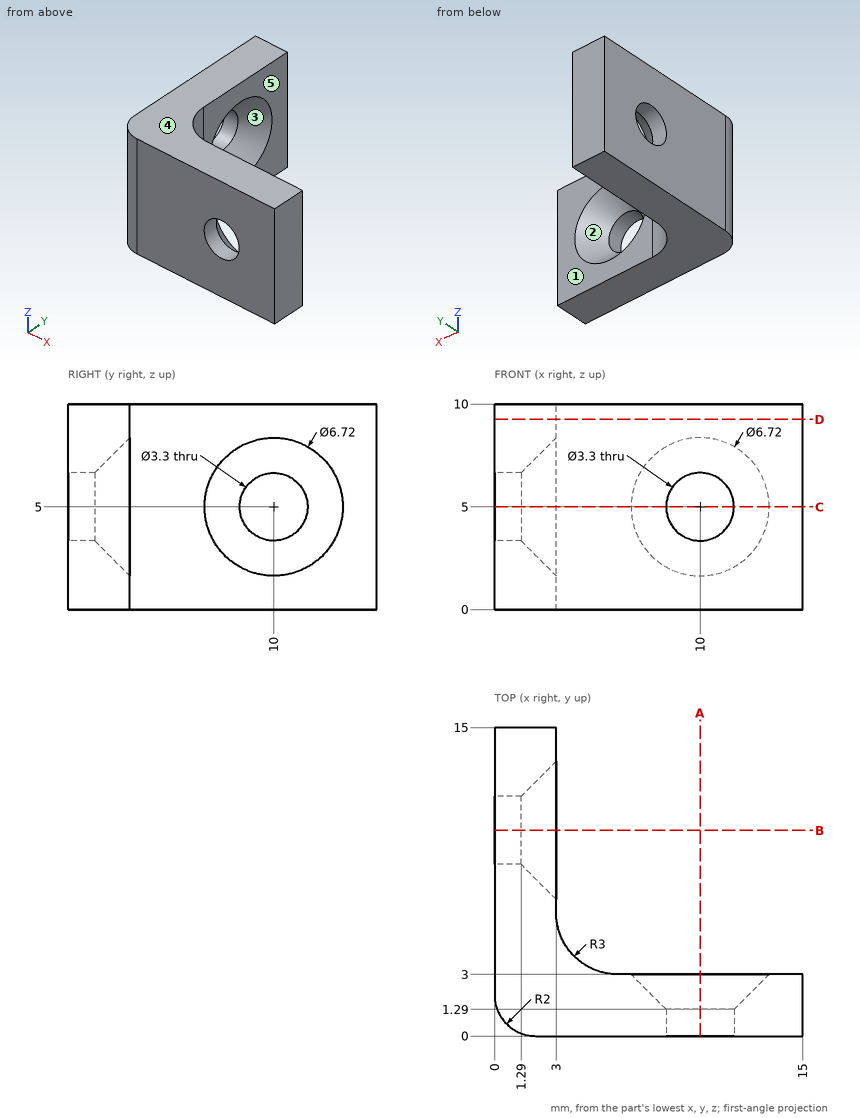
Job drawing, mm, ordinate dimensions from the low corner. One solid piece. A direction names the side the tool comes from. Coordinates: 2 decimals unless noted, no trailing zeros. Loops run counter-clockwise (first coordinate to the right, second up) from the corner with the lowest first, then second, coordinate; pieces in that order, holes last. Notation, with made-up numbers: (53.5, 47) - (100.5, 47) arc R15 ccw to (100.5, 52) - close; hole circle Ø3 at (46.25, 10). An arc over 180 degrees is marked (long way). Answer as a JSON object with one key per item and string values. Group by question number.
(1) Cut at A-A (x = 10). Give the cut face in (y, z), then the cut area to 3 significant figures.
(2) Cut at C-C (z = 5). Give the cut face in (x, y), then the cut area to 3 significant figures.
(3) Tool access for the marked faces 1 and 2: list every direction of +Z, -Z, +X, -X, +Y, -Y with a clear straight run to the whole face (end or side of a thin tool).
(4) Probe line 1 along Z through (x, y) = (10, 0.6); line 2 along X through (y, z) = (8.75, 7); line 3 along Y through (x, z) = (0.3, 5). List the from-to ranges inside material, lowest first.
(5) Cut at D-D (z = 9.25). Give the cut face in (x, y).
(6) Two-plate mould, pull along Z, no slides. Class the marked faces 3, 4 and 5: released by +Z, released by -Z, zero draft, split by the parting line, or undercut.
(7) Flat gauge pins, fed straight in: pin 1 (1.5 mm diameter, centred on y = 9, z = 4, fed in from +X); pin 2 (2.5 mm diameter, centred on x = 10.5, z = 6.5, fed in from +Y); pin 3 (3 mm diameter, centred on x = 6.5, z = 8.5, fed in from +Y). Where does each tip first touch, or does it go through?
Geometry says:
{
 "1": {"outline": "(0, 0) - (3, 0) - (3, 1.64) - (1.29, 3.35) - (0, 3.35) - close; (0, 6.65) - (1.29, 6.65) - (3, 8.36) - (3, 10) - (0, 10) - close", "area": "17.2 mm^2"},
 "2": {"outline": "(0, 2) arc R2 ccw to (2, 0) - (8.35, 0) - (8.35, 1.29) - (6.64, 3) - (6, 3) arc R3 cw to (3, 6) - (3, 6.64) - (1.29, 8.35) - (0, 8.35) - close; (0, 11.65) - (1.29, 11.65) - (3, 13.36) - (3, 15) - (0, 15) - close; (11.65, 0) - (15, 0) - (15, 3) - (13.36, 3) - (11.65, 1.29) - close", "area": "56.4 mm^2"},
 "3": {"face 1": "+Z, -Z, +X, +Y", "face 2": "+Y"},
 "4": {"line 1": "z = 0 to 3.35, 6.65 to 10", "line 2": "x = 0 to 2", "line 3": "y = 0.95 to 8.35, 11.65 to 15"},
 "5": {"outline": "(0, 2) arc R2 ccw to (2, 0) - (15, 0) - (15, 3) - (6, 3) arc R3 cw to (3, 6) - (3, 15) - (0, 15) - close"},
 "6": {"face 3": "undercut", "face 4": "released by +Z", "face 5": "zero draft"},
 "7": {"pin 1": "stops at x = 1.8", "pin 2": "stops at y = 2.47", "pin 3": "stops at y = 3.17"}
}
